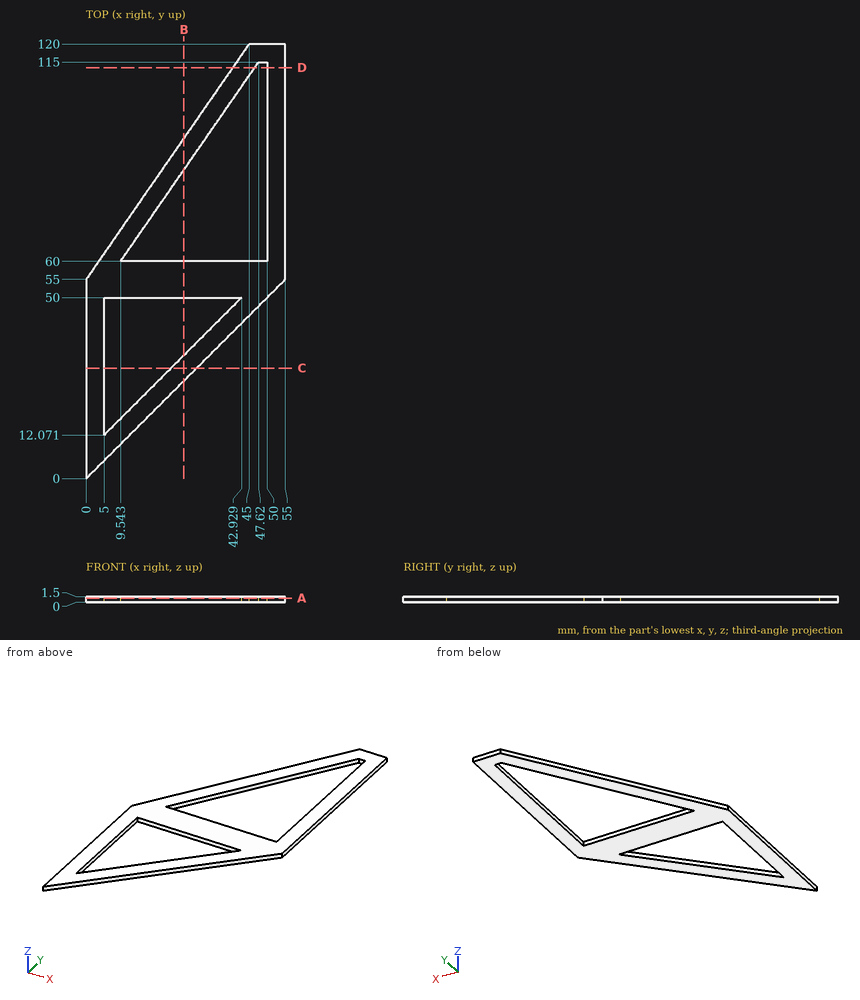
Could you check a few things on this drawing? It's one solid part, dimensions in mm from its lowest x, y, z. Coordinates: 2 decimals unless noted, no trailing zeros. Write each loop counter-clockwise with the first axis right and the second up, starting at its lowest first coordinate (ties: lowest second). Pieces come first, ordered by that corner, then holes. Notation, with made-up numbers: (49, -6.5) - (62, -6.5) arc R11 cw to (62, 8.5) - close; hole circle Ø1 at (28.5, 49). An arc over 180 degrees is marked (long way). Put each result on its own line as item: value. Start each with the question number.
Q1. I want a section at D-D on y = 113.5. Write out the boundary of the cut face in (x, z).
Q2. I want a section at C-C on y = 30.5. Write out the boundary of the cut face in (x, z), plus the area to 3 significant figures.
Q3. I want a section at B-B on x = 27. Write out the boundary of the cut face in (y, z).
Q4. Please list where these lines run through material, in increasing order: L1, parallel to Y at x = 14, z = 1.05; L2, parallel to Y at x = 30.5, z = 1.15 (1 decimal); L3, parallel to X at y = 111.5, z = 0.45 (1 decimal).
Q5. I want a section at A-A on z = 1.1. Write out the boundary of the cut face in (x, y), plus the area to 3 significant figures.
Checks:
1. outline: (40.5, 0) - (46.58, 0) - (46.58, 1.5) - (40.5, 1.5) - close; (50, 0) - (55, 0) - (55, 1.5) - (50, 1.5) - close
2. outline: (0, 0) - (5, 0) - (5, 1.5) - (0, 1.5) - close; (23.43, 0) - (30.5, 0) - (30.5, 1.5) - (23.43, 1.5) - close
2. area: 18.1 mm²
3. outline: (27, 0) - (34.07, 0) - (34.07, 1.5) - (27, 1.5) - close; (50, 0) - (60, 0) - (60, 1.5) - (50, 1.5) - close; (85.22, 0) - (94, 0) - (94, 1.5) - (85.22, 1.5) - close
4. L1: 14 to 21.07, 50 to 60, 66.44 to 75.22
4. L2: 30.5 to 37.6, 50 to 60, 90.3 to 99.1
4. L3: 39.1 to 45.2, 50 to 55
5. outline: (0, 0) - (55, 55) - (55, 120) - (45, 120) - (0, 55) - close; hole (5, 12.07) - (42.93, 50) - (5, 50) - close; hole (9.54, 60) - (50, 60) - (50, 115) - (47.62, 115) - close
5. area: 1,730 mm²
